Geometry: final body of the model. Coordinates: model frame, mm. Face numbers are marked on the shaded views. A direction names the side the tool comes from. Give positions to 0.01 mm unless a question says otherwise; leave off trailing zeros. Write each loop counter-clockwise with the first axis right and the second up, starting at its lowest first coordinate (ties: lowest second). Pieces come first, ordered by that corner, then holes.
```python
from build123d import *

# Parameters (mm, degrees)
EXTRUDE_1_DEPTH     = 5
CUT_EXTRUDE_1_DEPTH = 10
SKETCH_3_W          = 10
SKETCH_3_H          = 5
EXTRUDE_2_DEPTH     = 5
SKETCH_4_W          = 5
SKETCH_4_H          = 10
EXTRUDE_3_DEPTH     = 5
SKETCH_5_W          = 10
SKETCH_5_H          = 5
CUT_EXTRUDE_2_DEPTH = 1
SKETCH_6_W          = 5
SKETCH_6_H          = 10
CUT_EXTRUDE_3_DEPTH = 1
CUT_EXTRUDE_5_DEPTH = 5


with BuildPart() as part:
    # 草图1 → 凸台-拉伸1 (new body)
    with BuildSketch(Plane.XY):
        Polygon((0, 0), (30, 0), (30, 30), align=None)
    extrude(amount=EXTRUDE_1_DEPTH)

    # 草图2 → 切除-拉伸1 (cut)
    with BuildSketch(Plane.XY.offset(5)):
        Polygon((17.121320344, 12.878679656), (15, 15), (0, 0), align=None)
        Polygon((17.121320344, 12.878679656), (30, 30), (15, 15), align=None)
    extrude(amount=-CUT_EXTRUDE_1_DEPTH, mode=Mode.SUBTRACT)

    # 草图3 → 凸台-拉伸2 (add)
    with BuildSketch(Plane.XZ):
        with Locations((5, 2.5)):
            Rectangle(SKETCH_3_W, SKETCH_3_H)
    extrude(amount=EXTRUDE_2_DEPTH)

    # 草图4 → 凸台-拉伸3 (add)
    with BuildSketch(Plane(origin=(30, 0, 0), x_dir=(0, 0, -1), z_dir=(1, 0, 0))):
        with Locations((-2.5, 25)):
            Rectangle(SKETCH_4_W, SKETCH_4_H)
    extrude(amount=EXTRUDE_3_DEPTH)

    # 草图5 → 切除-拉伸2 (cut)
    with BuildSketch(Plane.XZ.offset(5)):
        with Locations((5, 2.5)):
            Rectangle(SKETCH_5_W, SKETCH_5_H)
    extrude(amount=-CUT_EXTRUDE_2_DEPTH, mode=Mode.SUBTRACT)

    # 草图6 → 切除-拉伸3 (cut)
    with BuildSketch(Plane(origin=(35, 0, 0), x_dir=(0, 0, -1), z_dir=(1, 0, 0))):
        with Locations((-2.5, 25)):
            Rectangle(SKETCH_6_W, SKETCH_6_H)
    extrude(amount=-CUT_EXTRUDE_3_DEPTH, mode=Mode.SUBTRACT)

    # 草图8 → 切除-拉伸5 (cut)
    with BuildSketch(Plane(origin=(-129.723125666, 239.943153128, 0), x_dir=(0, 1, 0), z_dir=(0, 0, -1))):
        with BuildLine():
            Line((-229.343153128, 156.723125666), (-229.343153128, 159.223125666))
            Line((-229.343153128, 159.223125666), (-229.343153128, 161.223125666))
            Line((-229.343153128, 161.223125666), (-226.543153128, 161.223125666))
            Line((-226.543153128, 161.223125666), (-226.543153128, 159.223125666))
            Line((-226.543153128, 159.223125666), (-226.543153128, 156.723125666))
            Line((-226.543153128, 156.723125666), (-225.493153128, 156.723125666))
            ThreePointArc((-225.493153128, 156.723125666), (-225.281021094, 156.6352577), (-225.193153128, 156.423125666))
            Line((-225.193153128, 156.423125666), (-225.193153128, 154.523125666))
            ThreePointArc((-225.193153128, 154.523125666), (-225.281021094, 154.310993631), (-225.493153128, 154.223125666))
            Line((-225.493153128, 154.223125666), (-226.593153128, 154.223125666))
            Line((-226.593153128, 154.223125666), (-226.593153128, 154.023125666))
            ThreePointArc((-226.593153128, 154.023125666), (-226.681021094, 153.810993631), (-226.893153128, 153.723125666))
            Line((-226.893153128, 153.723125666), (-228.993153128, 153.723125666))
            ThreePointArc((-228.993153128, 153.723125666), (-229.205285163, 153.810993631), (-229.293153128, 154.023125666))
            Line((-229.293153128, 154.023125666), (-229.293153128, 154.223125666))
            Line((-229.293153128, 154.223125666), (-230.393153128, 154.223125666))
            ThreePointArc((-230.393153128, 154.223125666), (-230.605285163, 154.310993631), (-230.693153128, 154.523125666))
            Line((-230.693153128, 154.523125666), (-230.693153128, 156.423125666))
            ThreePointArc((-230.693153128, 156.423125666), (-230.605285163, 156.6352577), (-230.393153128, 156.723125666))
            Line((-230.393153128, 156.723125666), (-229.343153128, 156.723125666))
        make_face()
        with BuildLine():
            Line((-239.443153128, 149.123125666), (-236.943153128, 149.123125666))
            Line((-236.943153128, 149.123125666), (-236.943153128, 150.173125666))
            ThreePointArc((-236.943153128, 150.173125666), (-236.855285163, 150.3852577), (-236.643153128, 150.473125666))
            Line((-236.643153128, 150.473125666), (-234.743153128, 150.473125666))
            ThreePointArc((-234.743153128, 150.473125666), (-234.531021094, 150.3852577), (-234.443153128, 150.173125666))
            Line((-234.443153128, 150.173125666), (-234.443153128, 149.073125666))
            Line((-234.443153128, 149.073125666), (-234.243153128, 149.073125666))
            ThreePointArc((-234.243153128, 149.073125666), (-234.031021094, 148.9852577), (-233.943153128, 148.773125666))
            Line((-233.943153128, 148.773125666), (-233.943153128, 146.673125666))
            ThreePointArc((-233.943153128, 146.673125666), (-234.031021094, 146.460993631), (-234.243153128, 146.373125666))
            Line((-234.243153128, 146.373125666), (-234.443153128, 146.373125666))
            Line((-234.443153128, 146.373125666), (-234.443153128, 145.273125666))
            ThreePointArc((-234.443153128, 145.273125666), (-234.531021094, 145.060993631), (-234.743153128, 144.973125666))
            Line((-234.743153128, 144.973125666), (-236.643153128, 144.973125666))
            ThreePointArc((-236.643153128, 144.973125666), (-236.855285163, 145.060993631), (-236.943153128, 145.273125666))
            Line((-236.943153128, 145.273125666), (-236.943153128, 146.323125666))
            Line((-236.943153128, 146.323125666), (-239.443153128, 146.323125666))
            Line((-239.443153128, 146.323125666), (-241.443153128, 146.323125666))
            Line((-241.443153128, 146.323125666), (-241.443153128, 149.123125666))
            Line((-241.443153128, 149.123125666), (-239.443153128, 149.123125666))
        make_face()
    extrude(amount=-CUT_EXTRUDE_5_DEPTH, mode=Mode.SUBTRACT)


solid = part.part
```
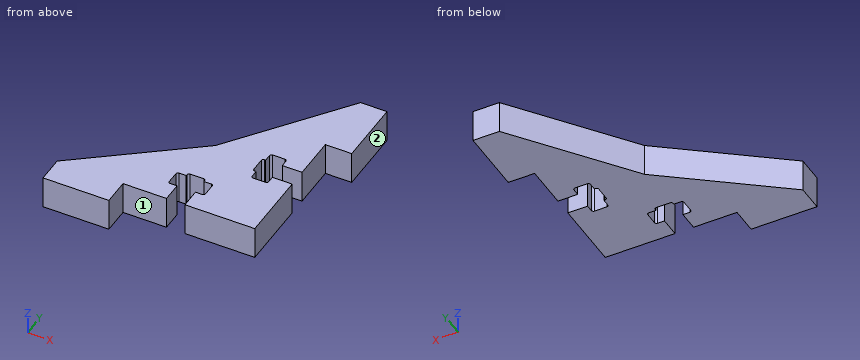
Item 1: Line query: L1, parallel to X at y = 10.5, z = 4.25; L2, parallel to Y at x = 28, z = 3.75; L3, parallel to Y at x = 20, z = 2.05. Output: solid intervals per line, ascending.
Found:
L1: x = 13.96 to 24.5, 27 to 30
L2: y = 0 to 10.6, 13.4 to 27.34
L3: y = 0 to 3, 5.5 to 16.71
Item 2: Pin query (flat end, axial travel): pin 1 Ø1.5 at (x, z) = (26, 3.5) entering from +Y; pin 2 Ø0.9 at (y, z) = (10.5, 3) entering from +X; pin 3 Ø1.5 at (y, z) = (21, 1.5) entering from -X. Return the tip coordinate at first contact, or that it passes through.
Found:
pin 1: stops at y = 25.68
pin 2: stops at x = 30
pin 3: stops at x = 22.67
Item 3: Section B-B, the plane y = 17.5. Return the cut outline in (x, z), plus the area to 3 significant figures.
Found:
outline: (20.6, 0) - (30, 0) - (30, 5) - (20.6, 5) - close
area: 47.0 mm2
Item 4: Reachability of the marked faces 1 and 2 from +Z, -Z, +X, -X, +Y, -Y: full face, straight path, thin tool, end or side. Return the list, or none.
Found:
face 1: +Z, -Z, +X, -Y
face 2: +Z, -Z, +X, +Y, -Y
Item 5: Section A-A, the plane x = 30.5. Return the cut outline in (y, z).
Found:
outline: (20, 0) - (30, 0) - (30, 5) - (20, 5) - close
